The listing builds one solid part. Answer for the finished solid, in the listing's coordinates (mm). Face numbers are marked on the shaded views. A direction names the side the tool comes from. Coordinates: 2 decimals unless noted, no trailing zeros. Order: outer loops, then holes, each group sorted by start corner. A loop starts at its lowest first (then second) coordinate and runs counter-clockwise, first axis right, second up. Notation, with made-up numbers: (66.5, 58) - (96.5, 58) arc R7 ccw to (96.5, 62) - close; hole circle Ø9 at (-20, 82). An arc over 180 degrees is marked (long way). Use a Markdown table: item, result. Add a question column.
Item 1: The part is cut by section B-B, the plane x = 4. Give the vertices of the cut face in (y, z).
Item 2: The part is cut by section A-A, the plane z = 19.5. Give the vertices of the cut face in (x, y), then the cut area to 3 significant figures.
Item 3: Find the intervals of material crossed by line 1 along Z through (x, y) = (-14.5, 5.5); line 2 along X through (y, z) = (3.25, 24.5); line 3 along Y through (x, z) = (13, 25.5), in increasing order.
Item 4: Flat-ended cylindrical pins translate along their axes: P1, Ø7, axis at y = -1, z = 28, coming from the -X side; P2, Ø10, axis at x = 13.5, y = 7, coming from the +Z side; P3, Ø1.5, axis at x = -8.5, y = -7, coming from the +Z side; P4, Ø4, axis at x = -10, y = -1.5, coming from the +Z side. Find the tip coordinate at first contact, or state that the pin passes through.
Item 5: For the marked faces 1 and 2, determine the directions among +Z, -Z, +X, -X, +Y, -Y from which every point of the face is accessible in a straight line to the end or side of a thin tool.
from build123d import *

# Parameters (mm, degrees)
SKETCH_1_W          = 38
SKETCH_1_H          = 18
EXTRUDE_1_DEPTH     = 4
EXTRUDE_3_DEPTH     = 34
CUT_EXTRUDE_1_DEPTH = 34


with BuildPart() as part:
    # 草图1 → 凸台-拉伸1 (new body)
    with BuildSketch(Plane.XY):
        Rectangle(SKETCH_1_W, SKETCH_1_H)
    extrude(amount=EXTRUDE_1_DEPTH)

    # 草图2 → 凸台-拉伸3 (add)
    with BuildSketch(Plane.XY.offset(4)):
        Polygon((19, 9), (19, -9), (-19, -9), (-19, -5), (15, -5), (15, 9), align=None)
    extrude(amount=EXTRUDE_3_DEPTH)

    # 草图4 → 切除-拉伸1 (cut)
    with BuildSketch(Plane(origin=(0, -5, 0), x_dir=(1, 0, 0), z_dir=(0, 1, 0))):
        Polygon((15, -38), (-19, -4), (-19, -38), align=None)
    extrude(amount=-CUT_EXTRUDE_1_DEPTH, mode=Mode.SUBTRACT)


solid = part.part
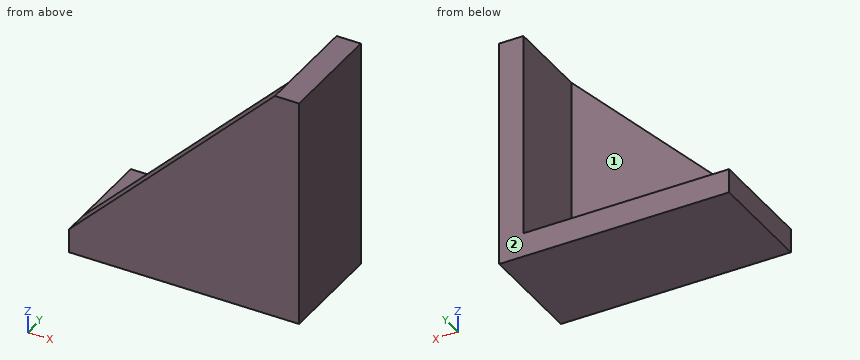
Solution:
| question | item | result |
|---|---|---|
| 1 | outline | (-9, 0) - (9, 0) - (9, 4) - (-5, 4) - (-5, 27) - (-9, 27) - close |
| 2 | outline | (-3.5, -9) - (19, -9) - (19, 9) - (15, 9) - (15, -5) - (-3.5, -5) - close |
| 2 | area | 146 mm2 |
| 3 | line 1 | z = 0 to 4 |
| 3 | line 2 | x = 15 to 19 |
| 3 | line 3 | y = -9 to -5 |
| 4 | P1 | stops at x = 15 |
| 4 | P2 | stops at z = 38 |
| 4 | P3 | stops at z = 15.25 |
| 4 | P4 | stops at z = 4 |
| 5 | face 1 | +Z, -X, +Y |
| 5 | face 2 | +Z, -Z, +X, -X, +Y |
